```python
from build123d import *

# Parameters (mm, degrees)
BOSS_EXTRUDE1_DEPTH = 15.875
SKETCH3_R           = 4.9022
CUT_EXTRUDE1_DEPTH  = 47.6627796
SKETCH4_W           = 46.0375
SKETCH4_H           = 19.05
CUT_EXTRUDE2_DEPTH  = 44.649033494
SKETCH5_R           = 3.2639
CUT_EXTRUDE3_DEPTH  = 4.7625
FILLET1_R           = 2.159


with BuildPart() as part:
    # Sketch1 → Boss-Extrude1 (new, symmetric)
    with BuildSketch(Plane.XY):
        with BuildLine():
            Line((-19.05, 12.7), (19.05, 12.7))
            Line((19.05, 12.7), (19.05, -12.7))
            Line((19.05, -12.7), (-19.05, -12.7))
            ThreePointArc((-19.05, -12.7), (-31.75, 0), (-19.05, 12.7))
        make_face()
    extrude(amount=BOSS_EXTRUDE1_DEPTH, both=True)

    # Sketch3 → Cut-Extrude1 (cut, through all)
    with BuildSketch(Plane.XY.offset(15.875)):
        with Locations((-19.05, 0)):
            Circle(SKETCH3_R)
    extrude(amount=-CUT_EXTRUDE1_DEPTH, mode=Mode.SUBTRACT)

    # Sketch4 → Cut-Extrude2 (cut, through all)
    with BuildSketch(Plane(origin=(0, 12.7, 0), x_dir=(1, 0, 0), z_dir=(0, 1, 0))):
        with Locations((-8.73125, 0)):
            Rectangle(SKETCH4_W, SKETCH4_H)
    extrude(amount=-CUT_EXTRUDE2_DEPTH, mode=Mode.SUBTRACT)

    # Sketch5 → Cut-Extrude3 (cut)
    with BuildSketch(Plane(origin=(19.05, 0, 0), x_dir=(0, 0, -1), z_dir=(1, 0, 0))):
        Circle(SKETCH5_R)
    extrude(amount=-CUT_EXTRUDE3_DEPTH, mode=Mode.SUBTRACT)

    # Fillet1
    fillet1_edges = [part.edges().sort_by_distance(p)[0] for p in [
        (19.05, 0, 15.875),
        (0, 12.7, 15.875),
        (-31.75, 0, 15.875),
        (0, 12.7, -15.875),
        (19.05, 0, -15.875),
        (0, -12.7, -15.875),
        (-31.75, 0, -15.875),
        (19.05, 12.7, 0),
        (19.05, -12.7, 0),
        (0, -12.7, 15.875),
    ]]
    fillet(fillet1_edges, radius=FILLET1_R)


solid = part.part
```
Geometry: final body of the model. Coordinates: model frame, mm. A direction names the side the tool comes from. Give positions to 0.01 mm unless a question says otherwise; leave off trailing zeros. Write each loop counter-clockwise with the first axis right and the second up, starting at its lowest first coordinate (ties: lowest second). Pieces come first, ordered by that corner, then holes.
1. Section query A-A, the plane z = 0. Return loops of the section in (x, y), then the cut area to 3 significant figures.
2. Draft query along X for faces 1 (the cylindrical face through (-31.747, -0.279, -11.591)), 2 (the cylindrical face through (-14.374, 1.472, -12.656)), 3 (the cylindrical face through (-14.374, 1.472, 12.744)), 4 (the cylindrical face through (-0.83, 12.08, -15.23)). Return one class per face: released by +X, released by -X, zero draft, split by the parting line, or undercut.
3. Pin query (flat end, axial travel): P1, Ø6, axis at y = -6, z = -10.5, coming from the -X side; P2, Ø5.5, axis at y = -1, z = 3.5, coming from the -X side. Return the tip coordinate at first contact, or that it passes through.
4. Section query C-C, the plane y = 0. Count the separate pieces of the cut face and the enclosed holes in it, then the cut area to 3 significant figures.
5. Section query D-D, the plane z = -12.5. Return loops of the section in (x, y).
6. Section query B-B, the plane x = 8.5. Return loops of the section in (y, z) (3 decimals).
7. Line query: probe 1 along Z at (x, y) = (-18.5, -10) (3 decimals); probe 2 along Y at (x, z) = (-19.05, 12); probe 3 along Y at (x, z) = (15.35, 0). Output: solid intervals per line, ascending.
8. Reachability of faces 5 (the flat face through (14.288, 3, -2)), 6 (the cylindrical face through (18.43, -0.15, -15.23)) from +Z, -Z, +X, -X, +Y, -Y: full face, straight path, thin tool, end or side. Return the list, or none.
Computed:
1. outline: (14.29, -12.7) - (16.89, -12.7) arc R2.16 ccw to (19.05, -10.54) - (19.05, -3.26) - (14.29, -3.26) - close; (14.29, 3.26) - (19.05, 3.26) - (19.05, 10.54) arc R2.16 ccw to (16.89, 12.7) - (14.29, 12.7) - close
1. area: 87.9 mm2
2. face 1: released by -X
2. face 2: undercut
2. face 3: undercut
2. face 4: zero draft
3. P1: stops at x = -31.39
3. P2: stops at x = 14.29
4. separate pieces: 4
4. enclosed holes: 0
4. area: 576 mm2
5. outline: (-19.05, -12.7) - (16.89, -12.7) arc R2.16 ccw to (19.05, -10.54) - (19.05, 10.54) arc R2.16 ccw to (16.89, 12.7) - (-19.05, 12.7) arc R12.7 ccw to start; hole circle Ø9.8 at (-19.05, 0)
6. outline: (-12.7, -13.716) arc R2.159 ccw to (-10.541, -15.875) - (10.541, -15.875) arc R2.159 ccw to (12.7, -13.716) - (12.7, -9.525) - (-12.7, -9.525) - close; (-12.7, 9.525) - (12.7, 9.525) - (12.7, 13.716) arc R2.159 ccw to (10.541, 15.875) - (-10.541, 15.875) arc R2.159 ccw to (-12.7, 13.716) - close
7. probe 1: z = -15.875 to -9.525, 9.525 to 15.875
7. probe 2: y = -12.7 to -4.9, 4.9 to 12.7
7. probe 3: y = -12.7 to -3.26, 3.26 to 12.7
8. face 5: -X, +Y, -Y
8. face 6: -Z, +X, +Y, -Y
